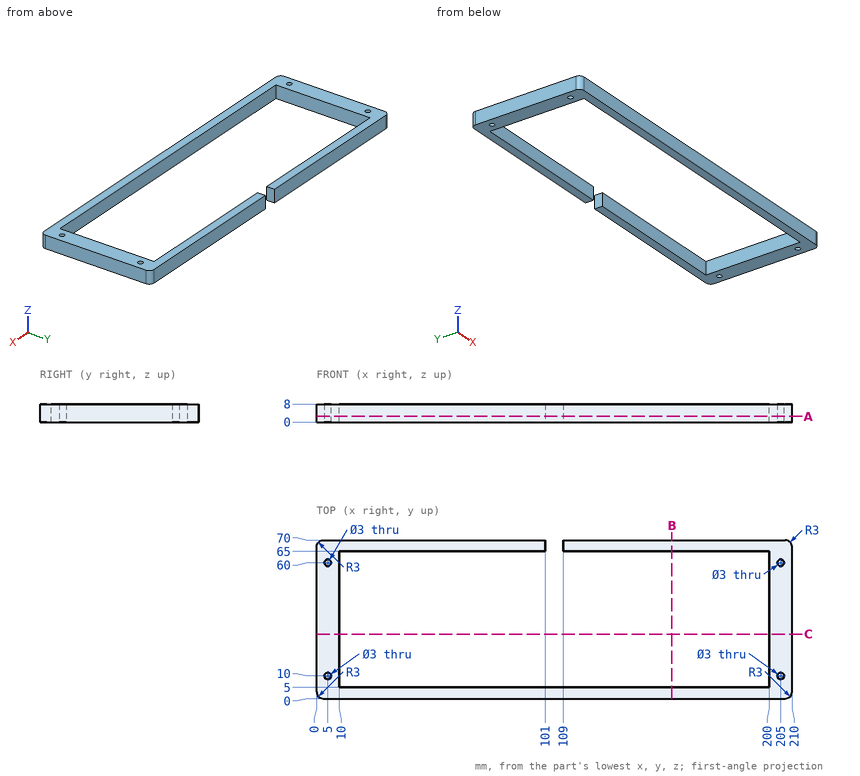
Verification items for this drawing (mm, ordinates from the low corner). Give positions to 0.01 mm unless a question says otherwise; leave off trailing zeros. Write each loop counter-clockwise with the first axis right and the second up, starting at its lowest first coordinate (ties: lowest second). Pieces come first, ordered by that corner, then holes.
1) Cross-section at B-B (x = 157). Record the boundary of the cut face in (y, z).
Values follow:
outline: (0, 0) - (5, 0) - (5, 8) - (0, 8) - close; (65, 0) - (70, 0) - (70, 8) - (65, 8) - close
2) Thickness scan on line 1 (X direction, y = 60, z = 6); line 2 (Y direction, x = 5, z = 4.5); line 3 (Y direction, x = 99.5, z = 6.5). Record the ranges inside material, lowest first.
Values follow:
line 1: x = 0 to 3.5, 6.5 to 10, 200 to 203.5, 206.5 to 210
line 2: y = 0 to 8.5, 11.5 to 58.5, 61.5 to 70
line 3: y = 0 to 5, 65 to 70
3) Go/stop test with flat-tipped pins: pin 1 Ø3.5 at (x, y) = (5, 10) entering from -Z; pin 2 Ø1.5 at (y, z) = (68.5, 4) entering from -X; pin 3 Ø2.5 at (y, z) = (68.5, 4) entering from +X. Record where each tip stops, or that it passes through.
Values follow:
pin 1: stops at z = 0
pin 2: stops at x = 0.1
pin 3: stops at x = 209.99
4) Cross-section at C-C (y = 28.5). Record the boundary of the cut face in (x, z).
Values follow:
outline: (0, 0) - (10, 0) - (10, 8) - (0, 8) - close; (200, 0) - (210, 0) - (210, 8) - (200, 8) - close
5) Cross-section at A-A (z = 2.5). Record the boundary of the cut face in (x, y), plus the area to 3 significant figures.
Values follow:
outline: (0, 3) arc R3 ccw to (3, 0) - (207, 0) arc R3 ccw to (210, 3) - (210, 67) arc R3 ccw to (207, 70) - (109, 70) - (109, 65) - (200, 65) - (200, 5) - (10, 5) - (10, 65) - (101, 65) - (101, 70) - (3, 70) arc R3 ccw to (0, 67) - close; hole circle Ø3 at (5, 10); hole circle Ø3 at (5, 60); hole circle Ø3 at (205, 10); hole circle Ø3 at (205, 60)
area: 3,220 mm2
